For this review, take the finished solid that the model builds, in its own axes (mm). Coordinates: 2 decimals unless noted, no trailing zeros. Loops run counter-clockwise (first coordinate to the right, second up) from the corner with the lowest first, then second, coordinate; pieces in that order, holes last. Notation, with made-up numbers: (-40, -25) -> (-34, -25) arc R18 ccw to (-34, 1) -> close; hole circle Ø2 at (-27.75, -34.75). An arc over 180 degrees is marked (long way). One line per item, written item: value.
from build123d import *

# Parameters (mm, degrees)
SKETCH1_W            = 218.44
SKETCH1_H            = 190.5
BOSS_EXTRUDE1_DEPTH  = 9.525
SKETCH2_W            = 206.375
SKETCH2_H            = 180.975
CUT_EXTRUDE1_DEPTH   = 9.525
SKETCH3_R            = 4.8895
CUT_EXTRUDE2_DEPTH   = 239.49386098
SKETCH4_W            = 12.7
SKETCH4_H            = 12.7
BOSS_EXTRUDE2_DEPTH  = 3.175
SKETCH5_R            = 1.27
CUT_EXTRUDE3_DEPTH   = 154.69623743
FILLET1_R            = 6.35
FILLET2_R            = 2.54
FILLET1_OF_MIRROR1_R = 6.35
FILLET2_OF_MIRROR1_R = 2.54
SKETCH6_W            = 12.7
SKETCH6_H            = 12.7
SKETCH6_R            = 1.27
BOSS_EXTRUDE3_DEPTH  = 3.175
FILLET3_R            = 2.54
FILLET4_R            = 6.35
FILLET3_OF_MIRROR7_R = 2.54
FILLET4_OF_MIRROR7_R = 6.35


with BuildPart() as part:
    # Sketch1 → Boss-Extrude1 (new body)
    with BuildSketch(Plane.XY):
        Rectangle(SKETCH1_W, SKETCH1_H)
    extrude(amount=BOSS_EXTRUDE1_DEPTH)

    # Sketch2 → Cut-Extrude1 (cut)
    with BuildSketch(Plane.XY.offset(9.525)):
        Rectangle(SKETCH2_W, SKETCH2_H)
    extrude(amount=-CUT_EXTRUDE1_DEPTH, mode=Mode.SUBTRACT)

    # Sketch3 → Cut-Extrude2 (cut, through all)
    with BuildSketch(Plane(origin=(109.22, 0, 0), x_dir=(0, 0, -1), z_dir=(1, 0, 0))):
        Circle(SKETCH3_R)
        with Locations((0, 57.404)):
            Circle(SKETCH3_R)
        with Locations((0, -57.404)):
            Circle(SKETCH3_R)
    extrude(amount=-CUT_EXTRUDE2_DEPTH, mode=Mode.SUBTRACT)

    # Sketch4 → Boss-Extrude2 (add)
    with BuildSketch(Plane(origin=(0, 0, 0), x_dir=(-1, 0, 0), z_dir=(0, 0, -1))):
        with Locations((-102.87, 101.6)):
            Rectangle(SKETCH4_W, SKETCH4_H)
    boss_extrude2 = extrude(amount=-BOSS_EXTRUDE2_DEPTH)

    # Sketch5 → Cut-Extrude3 (cut, through all)
    with BuildSketch(Plane.XY.offset(3.175)):
        with Locations((102.87, 101.6)):
            Circle(SKETCH5_R)
    cut_extrude3 = extrude(amount=-CUT_EXTRUDE3_DEPTH, mode=Mode.SUBTRACT)

    # Fillet1
    fillet1_edges = [part.edges().sort_by_distance(p)[0] for p in [
        (96.52, 107.95, 1.5875),
        (109.22, 107.95, 1.5875),
    ]]
    fillet(fillet1_edges, radius=FILLET1_R - 0.0001)  # a hair under: the kernel refuses the full size

    # Fillet2
    fillet2_edges = [part.edges().sort_by_distance(p)[0] for p in [
        (102.87, 95.25, 3.175),
        (96.52, 95.25, 1.5875),
    ]]
    fillet(fillet2_edges, radius=FILLET2_R)

    # Mirror1: Boss-Extrude2, Cut-Extrude3 across plane
    add(boss_extrude2.mirror(Plane(origin=(0, 0, 0), x_dir=(0, 0, 1), z_dir=(1, 0, 0))))
    add(cut_extrude3.mirror(Plane(origin=(0, 0, 0), x_dir=(0, 0, 1), z_dir=(1, 0, 0))), mode=Mode.SUBTRACT)

    # Fillet1 of Mirror1
    fillet1_of_mirror1_edges = [part.edges().sort_by_distance(p)[0] for p in [
        (-96.52, 107.95, 1.5875),
        (-109.22, 107.95, 1.5875),
    ]]
    fillet(fillet1_of_mirror1_edges, radius=FILLET1_OF_MIRROR1_R - 0.0001)  # a hair under: the kernel refuses the full size

    # Fillet2 of Mirror1
    fillet2_of_mirror1_edges = [part.edges().sort_by_distance(p)[0] for p in [
        (-102.87, 95.25, 3.175),
        (-96.52, 95.25, 1.5875),
    ]]
    fillet(fillet2_of_mirror1_edges, radius=FILLET2_OF_MIRROR1_R)

    # Sketch6 → Boss-Extrude3 (add)
    with BuildSketch(Plane(origin=(0, 0, 0), x_dir=(-1, 0, 0), z_dir=(0, 0, -1))):
        with Locations((-102.87, -101.6)):
            Rectangle(SKETCH6_W, SKETCH6_H)
        with Locations((-102.87, -101.6)):
            Circle(SKETCH6_R, mode=Mode.SUBTRACT)
    boss_extrude3 = extrude(amount=-BOSS_EXTRUDE3_DEPTH)

    # Fillet3
    fillet3_edges = [part.edges().sort_by_distance(p)[0] for p in [
        (102.87, -95.25, 3.175),
        (96.52, -95.25, 1.5875),
    ]]
    fillet(fillet3_edges, radius=FILLET3_R)

    # Fillet4
    fillet4_edges = [part.edges().sort_by_distance(p)[0] for p in [
        (109.22, -107.95, 1.5875),
        (96.52, -107.95, 1.5875),
    ]]
    fillet(fillet4_edges, radius=FILLET4_R - 0.0001)  # a hair under: the kernel refuses the full size

    # Mirror7: Boss-Extrude3 across plane
    add(boss_extrude3.mirror(Plane(origin=(0, 0, 0), x_dir=(0, 0, 1), z_dir=(1, 0, 0))))

    # Fillet3 of Mirror7
    fillet3_of_mirror7_edges = [part.edges().sort_by_distance(p)[0] for p in [
        (-102.87, -95.25, 3.175),
        (-96.52, -95.25, 1.5875),
    ]]
    fillet(fillet3_of_mirror7_edges, radius=FILLET3_OF_MIRROR7_R)

    # Fillet4 of Mirror7
    fillet4_of_mirror7_edges = [part.edges().sort_by_distance(p)[0] for p in [
        (-109.22, -107.95, 1.5875),
        (-96.52, -107.95, 1.5875),
    ]]
    fillet(fillet4_of_mirror7_edges, radius=FILLET4_OF_MIRROR7_R - 0.0001)  # a hair under: the kernel refuses the full size


solid = part.part
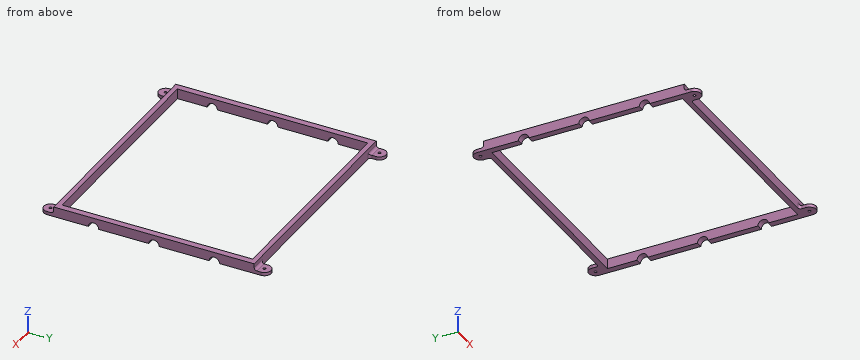
1. To check wall thickness, follow probe 1 along Y at (x, z) = (102.87, 1.35); probe 2 along X at (y, z) = (101.6, 1.9); probe 3 along Y at (x, z) = (-76, 5.5). State the ranges of each line that lie inside material, in increasing order. Write a range as from..to.
Return value:
probe 1: y = -107.95..-102.87, -100.33..-90.49, 90.49..100.33, 102.87..107.95
probe 2: x = -109.22..-104.14, -101.6..-96.52, 96.52..101.6, 104.14..109.22
probe 3: y = -95.25..-90.49, 90.49..95.25
2. Insertion check: pin 1 Ø1.5 at (x, y) = (-102.87, -101.6) entering from +Z; pin 2 Ø8 at (x, y) = (104.5, 100.5) entering from +Z; pin 3 Ø2 at (x, z) = (-41.5, 2.5) entering from -Y; pin 4 Ø8 at (x, y) = (-101.5, -104) entering from +Z (3 decimals). Each pin has a flat end and moves straight along its axis. Give the tip position at first contact, or say it passes through.
Return value:
pin 1: passes through
pin 2: stops at z = 3.53
pin 3: stops at y = -95.25
pin 4: stops at z = 3.175
3. Take a section at B-B, the plane y = 0. Give the boundary of the cut face in (x, z) (1 decimal), and give its area (3 significant figures).
Return value:
outline: (-109.2, 4.9) -> (-103.2, 4.9) -> (-103.2, 9.5) -> (-109.2, 9.5) -> close; (103.2, 4.9) -> (109.2, 4.9) -> (109.2, 9.5) -> (103.2, 9.5) -> close
area: 55.9 mm2
